Geometry check sheet. Reference: the model listing, model coordinates, mm. Face numbers are marked on the shaded views. A direction names the side the tool comes from. Give positions to 0.01 mm unless a question says otherwise; leave off trailing zeros. Loops run counter-clockwise (first coordinate to the right, second up) from the corner with the lowest first, then second, coordinate; pieces in that order, holes last. Notation, with made-up numbers: (48.5, -24) -> (100.5, -24) arc R23 cw to (100.5, 3) -> close; hole circle Ø8 at (52.25, 11). An arc over 180 degrees is marked (long way). Write item = value, one per line. Start each with the question number.
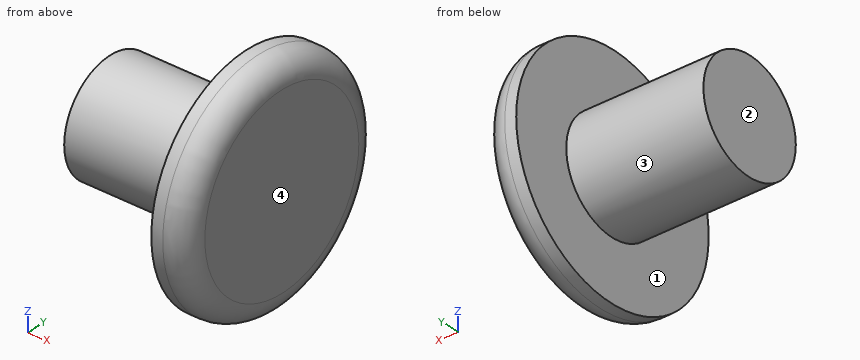
```python
from build123d import *

# Parameters (mm, degrees)
F0_R     = 5
F1_DEPTH = 1.5
F2_R     = 1
F3_R     = 2.4
F4_DEPTH = 6


with BuildPart() as f1:
    # F0 (on Right) → F1 (new body)
    with BuildSketch(Plane.YZ):
        Circle(F0_R)
    extrude(amount=-F1_DEPTH)

    # F2
    f2_edges = [f1.edges().sort_by_distance(p)[0] for p in [
        (0, -5, 0),
    ]]
    fillet(f2_edges, radius=F2_R)

    # F3 (on face) → F4 (join)
    with BuildSketch(Plane(origin=(-1.5, 0, 0), x_dir=(0, -1, 0), z_dir=(-1, 0, 0))):
        Circle(F3_R)
    extrude(amount=F4_DEPTH)


solid = f1.part
```
1) Draft check along Y on the marked faces 3 and 4. Enter one of: released by +Y, released by -Y, zero draft, split by the parting line, or undercut.
2) Tool access check on the marked faces 1 and 2. Record the directions out of +Z, -Z, +X, -X, +Y, -Y that give a thin tool (end or side, any length) a straight path to the whole face; none if there is none.
3) Thickness scan on line 1 (X direction, y = 2, z = 1.75); line 2 (X direction, y = -4, z = -2); line 3 (Z direction, x = -5, y = 0.5). Record the ranges inside material, lowest first.
4) Section check A-A (z = 0). Enter the section's corners in (x, y).
5) Depth check by flat-ended pin: pin 1 Ø3 at (x, z) = (-6.5, -3.5) entering from +Y; pin 2 Ø4 at (x, z) = (-3, -3) entering from +Y. Enter the tip coordinate at first touch or a pass-through.
6) Section check C-C (x = -2.5). Enter the section's corners in (y, z), plus the area to 3 significant figures.
Check result:
q1.face_3 = split by the parting line
q1.face_4 = zero draft
q2.face_1 = -X
q2.face_2 = +Z, -Z, -X, +Y, -Y
q3.line_1 = -1.5 to 0
q3.line_2 = -1.5 to -0.12
q3.line_3 = -2.35 to 2.35
q4.outline = (-7.5, -2.4) -> (-1.5, -2.4) -> (-1.5, -5) -> (-1, -5) arc R1 ccw to (0, -4) -> (0, 4) arc R1 ccw to (-1, 5) -> (-1.5, 5) -> (-1.5, 2.4) -> (-7.5, 2.4) -> close
q5.pin_1 = 1.33
q5.pin_2 = 4.71
q6.outline = circle Ø4.8 at (0, 0)
q6.area = 18.1 mm2
